Could you check a few things on this model? Use its own coordinates, in mm. Round coordinates to 2 decimals unless told otherwise and drop trailing zeros. Order: outer loops, then holes, each group sorted by start corner. A loop starts at its lowest first (then second) coordinate and runs counter-clockwise, first axis right, second up.
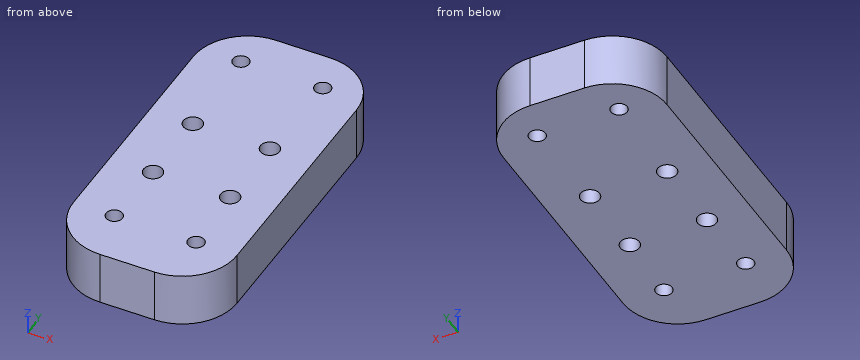
```python
from build123d import *

# Parameters (mm, degrees)
SKETCH_1_W      = 30
SKETCH_1_H      = 62.5
SKETCH_1_R      = 1.75
SKETCH_1_R_2    = 1.5
EXTRUDE_1_DEPTH = 10
FILLET_1_R      = 10


with BuildPart() as part:
    # 草图1 → 凸台-拉伸1 (new body)
    with BuildSketch(Plane.XY):
        with Locations((0, 1.25)):
            Rectangle(SKETCH_1_W, SKETCH_1_H)
        with Locations((7.071067812, 7.071067812)):
            Circle(SKETCH_1_R, mode=Mode.SUBTRACT)
        with Locations((-7.071067812, 7.071067812)):
            Circle(SKETCH_1_R, mode=Mode.SUBTRACT)
        with Locations((7.071067812, -7.071067812)):
            Circle(SKETCH_1_R, mode=Mode.SUBTRACT)
        with Locations((-7.071067812, -7.071067812)):
            Circle(SKETCH_1_R, mode=Mode.SUBTRACT)
        with Locations((7.5, 25)):
            Circle(SKETCH_1_R_2, mode=Mode.SUBTRACT)
        with Locations((-7.5, 25)):
            Circle(SKETCH_1_R_2, mode=Mode.SUBTRACT)
        with Locations((7.5, -20)):
            Circle(SKETCH_1_R_2, mode=Mode.SUBTRACT)
        with Locations((-7.5, -20)):
            Circle(SKETCH_1_R_2, mode=Mode.SUBTRACT)
    extrude(amount=EXTRUDE_1_DEPTH)

    # 圆角1
    fillet_1_edges = [part.edges().sort_by_distance(p)[0] for p in [
        (15, -30, 5),
        (-15, -30, 5),
        (-15, 32.5, 5),
        (15, 32.5, 5),
    ]]
    fillet(fillet_1_edges, radius=FILLET_1_R)


solid = part.part
```
Q1. Imagine slicing it at B-B, the plane x = 8. Please give me the cut outline in (y, z).
Q2. Imagine slicing it at D-D, the plane x = -7.5. Please give me the cut outline in (y, z).
Q3. Imagine slicing it at C-C, the plane z = 7.75. State how many separate pieces and enclosed holes the cut face has, then the cut area to 3 significant figures.
Q4. I need wall thicknesses on L1, parallel to X at y = 7, z = 4.75; L2, parallel to X at y = 6, z = 8.25; L3, parallel to Y at x = -6.5, z = 0.5. Which ranges of each line are inside material? Lowest first, please.
Q5. For P1, Ø4.5, axis at x = 7.07, y = 7.07, coming from the +Z side; P2, Ø4, axis at x = -12, z = 5, coming from the -Y side, each with a flat end and sliding along its axis, tell me the tip position at first contact or that it passes through.
Q6. Imagine slicing it at A-A, the plane y = 25. Please give me the cut outline in (x, z), then the cut area to 3 significant figures.
Filled in:
1. outline: (-29.54, 0) - (-21.41, 0) - (-21.41, 10) - (-29.54, 10) - close; (-18.59, 0) - (-8.55, 0) - (-8.55, 10) - (-18.59, 10) - close; (-5.59, 0) - (5.59, 0) - (5.59, 10) - (-5.59, 10) - close; (8.55, 0) - (23.59, 0) - (23.59, 10) - (8.55, 10) - close; (26.41, 0) - (32.04, 0) - (32.04, 10) - (26.41, 10) - close
2. outline: (-29.68, 0) - (-21.5, 0) - (-21.5, 10) - (-29.68, 10) - close; (-18.5, 0) - (-8.77, 0) - (-8.77, 10) - (-18.5, 10) - close; (-5.37, 0) - (5.37, 0) - (5.37, 10) - (-5.37, 10) - close; (8.77, 0) - (23.5, 0) - (23.5, 10) - (8.77, 10) - close; (26.5, 0) - (32.18, 0) - (32.18, 10) - (26.5, 10) - close
3. separate pieces: 1
3. enclosed holes: 8
3. area: 1,720 mm2
4. L1: x = -15 to -8.82, -5.32 to 5.32, 8.82 to 15
4. L2: x = -15 to -8.46, -5.69 to 5.69, 8.46 to 15
4. L3: y = -29.89 to -21.12, -18.88 to -8.73, -5.42 to 5.42, 8.73 to 23.88, 26.12 to 32.39
5. P1: stops at z = 10
5. P2: stops at y = -28.66
6. outline: (-14.68, 0) - (-9, 0) - (-9, 10) - (-14.68, 10) - close; (-6, 0) - (6, 0) - (6, 10) - (-6, 10) - close; (9, 0) - (14.68, 0) - (14.68, 10) - (9, 10) - close
6. area: 234 mm2
